Here's the drawing with two shaded views (mm, measured from the low corner). I have some questions. Round coordinates to 2 decimals unless told otherwise and drop trailing zeros. Order: outer loops, then holes, each group sorted by start corner. A loop starts at its lowest first (then second) coordinate and runs counter-clockwise, first axis right, second up.
Q1. If I drill on line 1 (Y direction, x = 4, z = 28.5) (1 decimal); line 2 (Z direction, x = 4, y = 5.5); line 3 (Y direction, x = 5, z = 32) (1 decimal), over which ranges is the centre line in solid material (lowest first)?
Q2. If we section it at D-D (x = 4): Please give me the cut outline in (y, z) (1 decimal).
Q3. If we section it at B-B (x = 6): Please give me the cut outline in (y, z) (1 decimal).
Q4. If we section it at A-A (y = 3): Please give me the cut outline in (x, z), plus the area to 3 significant figures.
Q5. Will these pins go through, and if not, where does the flat tip stop? P1, Ø2, axis at y = 6.5, z = 29, coming from the +X side; P2, Ø3, axis at y = 2, z = 29.5, coming from the +X side.
Q6. If we section it at C-C (z = 23.5): Please give me the cut outline in (x, y) (1 decimal).
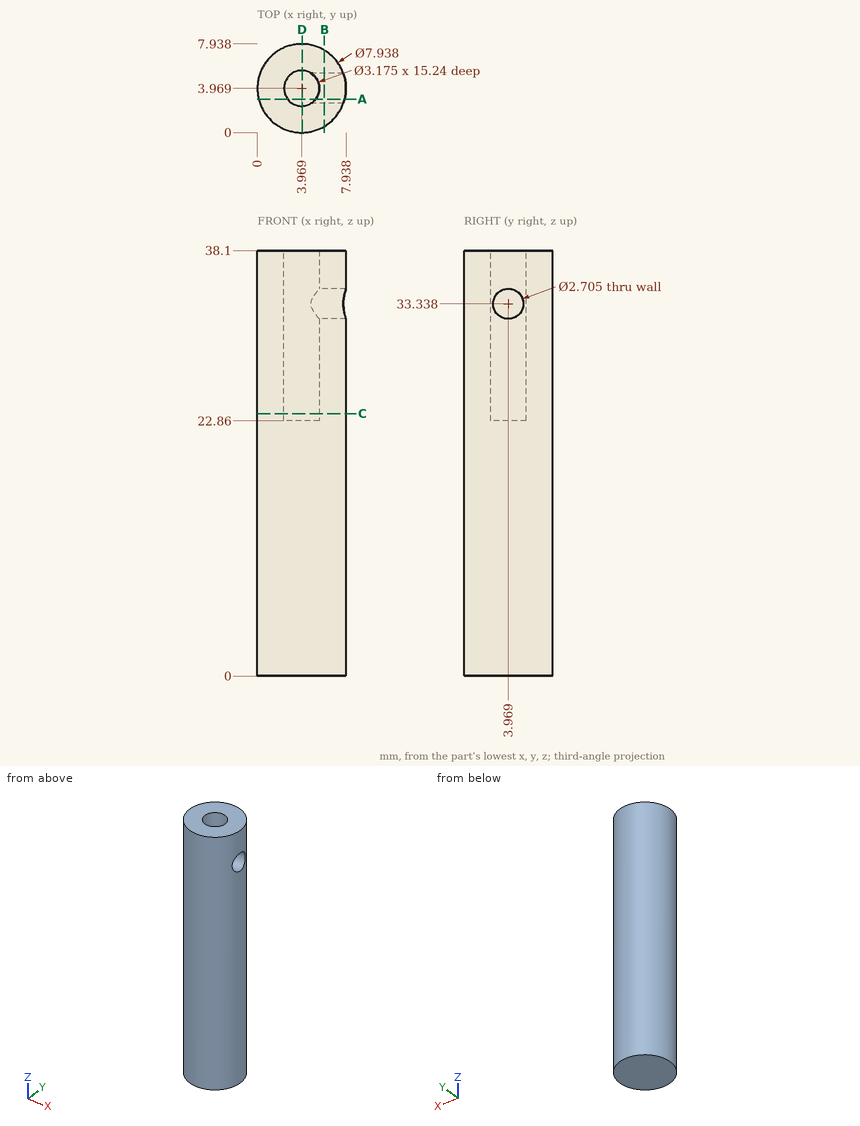
Solution:
1. line 1: y = 0 to 2.4, 5.6 to 7.9
1. line 2: z = 0 to 22.86
1. line 3: y = 0.1 to 2.8, 5.2 to 7.8
2. outline: (0, 0) - (7.9, 0) - (7.9, 38.1) - (5.6, 38.1) - (5.6, 22.9) - (2.4, 22.9) - (2.4, 38.1) - (0, 38.1) - close
3. outline: (0.6, 0) - (7.4, 0) - (7.4, 38.1) - (0.6, 38.1) - close; hole circle Ø2.7 at (4, 33.3)
4. outline: (0.12, 0) - (7.82, 0) - (7.82, 32.39) - (5.23, 32.39) - (5.23, 22.86) - (2.71, 22.86) - (2.71, 38.1) - (0.12, 38.1) - close; (5.23, 34.28) - (7.82, 34.28) - (7.82, 38.1) - (5.23, 38.1) - close
4. area: 250 mm2
5. P1: stops at x = 7.63
5. P2: stops at x = 7.91
6. outline: circle Ø7.9 at (4, 4); hole circle Ø3.2 at (4, 4)
